Verification items for the finished model (mm, model axes). A direction names the side the tool comes from. Give positions to 0.01 mm unless a question says otherwise; leave off trailing zeros. Order: outer loops, then holes, each group sorted by start corner. A loop starts at its lowest first (then second) coordinate and runs counter-clockwise, first axis right, second up.
from build123d import *

# Parameters (mm, degrees)
SKETCH1_W           = 40
SKETCH1_H           = 45
BOSS_EXTRUDE1_DEPTH = 9.09
SKETCH2_R           = 1.5
CUT_EXTRUDE1_DEPTH  = 32.44643223
SKETCH3_R           = 9.25
CUT_EXTRUDE4_DEPTH  = 2.5
SKETCH4_R           = 4
CUT_EXTRUDE5_DEPTH  = 31.816847665
SKETCH5_W           = 40
SKETCH5_H           = 59.09
BOSS_EXTRUDE2_DEPTH = 7.35
SKETCH6_R           = 1.7
CUT_EXTRUDE6_DEPTH  = 77.919621034
FILLET1_R           = 4


with BuildPart() as part:
    # Sketch1 → Boss-Extrude1 (new body)
    with BuildSketch(Plane(origin=(0, 0, 0), x_dir=(0, 1, 0), z_dir=(0, 0, 1))):
        Rectangle(SKETCH1_W, SKETCH1_H)
    extrude(amount=BOSS_EXTRUDE1_DEPTH)

    # Sketch2 → Cut-Extrude1 (cut, through all)
    with BuildSketch(Plane.XY.offset(9.09)):
        with Locations((0, 11)):
            Circle(SKETCH2_R)
        with Locations((11, 0)):
            Circle(SKETCH2_R)
        with Locations((0, -11)):
            Circle(SKETCH2_R)
        with Locations((-11, 0)):
            Circle(SKETCH2_R)
    extrude(amount=-CUT_EXTRUDE1_DEPTH, mode=Mode.SUBTRACT)

    # Sketch3 → Cut-Extrude4 (cut)
    with BuildSketch(Plane.XY.offset(9.09)):
        Circle(SKETCH3_R)
    extrude(amount=-CUT_EXTRUDE4_DEPTH, mode=Mode.SUBTRACT)

    # Sketch4 → Cut-Extrude5 (cut, through all)
    with BuildSketch(Plane.XY.offset(6.59)):
        Circle(SKETCH4_R)
    extrude(amount=-CUT_EXTRUDE5_DEPTH, mode=Mode.SUBTRACT)

    # Sketch5 → Boss-Extrude2 (add)
    with BuildSketch(Plane(origin=(-22.5, 0, 0), x_dir=(0, -1, 0), z_dir=(-1, 0, 0))):
        with Locations((0, 29.545)):
            Rectangle(SKETCH5_W, SKETCH5_H)
    extrude(amount=BOSS_EXTRUDE2_DEPTH)

    # Sketch6 → Cut-Extrude6 (cut, through all)
    with BuildSketch(Plane.YZ.offset(-22.5)):
        with Locations(Location((-10, 49.09, 0), (0, 0, 270))):
            Circle(SKETCH6_R)
        with Locations(Location((10, 49.09, 0), (0, 0, 270))):
            Circle(SKETCH6_R)
        with Locations(Location((-10, 24.09, 0), (0, 0, 270))):
            Circle(SKETCH6_R)
        with Locations(Location((10, 24.09, 0), (0, 0, 270))):
            Circle(SKETCH6_R)
    extrude(amount=-CUT_EXTRUDE6_DEPTH, mode=Mode.SUBTRACT)

    # Fillet1
    fillet1_edges = [part.edges().sort_by_distance(p)[0] for p in [
        (-22.5, 0, 9.09),
    ]]
    fillet(fillet1_edges, radius=FILLET1_R)


solid = part.part
(1) Section check A-A, the plane x = 11. Enter the section's corners in (y, z), then the cut area to 3 significant figures.
Solved:
outline: (-20, 0) - (-1.5, 0) - (-1.5, 9.09) - (-20, 9.09) - close; (1.5, 0) - (20, 0) - (20, 9.09) - (1.5, 9.09) - close
area: 336 mm2
(2) Scan lines: line 1 (Y direction, x = 0, z = 6); line 2 (Y direction, x = -27, z = 24); line 3 (X direction, y = 6.5, z = 53.5). Record each from-to range of solid material in increasing order.
Solved:
line 1: y = -20 to -12.5, -9.5 to -4, 4 to 9.5, 12.5 to 20
line 2: y = -20 to -11.7, -8.3 to 8.3, 11.7 to 20
line 3: x = -29.85 to -22.5
(3) Set-up check for faces 1 (the cylindrical face through (-26.12, -10.65, 22.52)), 2 (the flat face through (6, -9, 9.09)), 3 (the cylindrical face through (-2.01, -9.03, 7.86)): record each of +Z, -Z, +X, -X, +Y, -Y from which the full face is reachable in a straight line by a thin tool's end or side.
Solved:
face 1: +X, -X
face 2: +Z, +X, +Y, -Y
face 3: +Z
(4) Release check for a two-part mould opening along Y. For faces 4 (the flat face through (-22.5, 0, 36)), 5 (the flat face through (-23, 20, 18)), 6 (the cylindrical face through (-12.5, 0.07, 4.61)) record: pulls with the +Y half, pulls with the -Y half, needs draft (parallel to the pull), parting line crosses it, or undercut.
Solved:
face 4: needs draft
face 5: pulls with the +Y half
face 6: undercut
(5) Section check B-B, the plane z = 49.09. Enter the section's corners in (x, y).
Solved:
outline: (-29.85, -20) - (-22.5, -20) - (-22.5, -11.7) - (-29.85, -11.7) - close; (-29.85, -8.3) - (-22.5, -8.3) - (-22.5, 8.3) - (-29.85, 8.3) - close; (-29.85, 11.7) - (-22.5, 11.7) - (-22.5, 20) - (-29.85, 20) - close
(6) Section check C-C, the plane y = 0. Enter the section's corners in (x, z).
Solved:
outline: (-29.85, 0) - (-12.5, 0) - (-12.5, 9.09) - (-18.5, 9.09) arc R4 cw to (-22.5, 13.09) - (-22.5, 59.09) - (-29.85, 59.09) - close; (-9.5, 0) - (-4, 0) - (-4, 6.59) - (-9.25, 6.59) - (-9.25, 9.09) - (-9.5, 9.09) - close; (4, 0) - (9.5, 0) - (9.5, 9.09) - (9.25, 9.09) - (9.25, 6.59) - (4, 6.59) - close; (12.5, 0) - (22.5, 0) - (22.5, 9.09) - (12.5, 9.09) - close
(7) Section check D-D, the plane y = -15.5. Enter the section's corners in (x, z).
Solved:
outline: (-29.85, 0) - (22.5, 0) - (22.5, 9.09) - (-18.5, 9.09) arc R4 cw to (-22.5, 13.09) - (-22.5, 59.09) - (-29.85, 59.09) - close
(8) Go/stop test with flat-tipped pins: pin 1 (12 mm diameter, centred on x = 0.5, y = -6.5, fed in from +Z); pin 2 (7 mm diameter, centred on x = 0, y = 0, fed in from +Z) (1 decimal); pin 3 (4 mm diameter, centred on y = -10, z = 24.09, fed in from +X); pin 4 (2 mm diameter, centred on x = -3, y = 0.5, fed in from +Z). Record where each tip stops, or that it passes through.
Solved:
pin 1: stops at z = 9.09
pin 2: passes through
pin 3: stops at x = -22.5
pin 4: stops at z = 6.59
